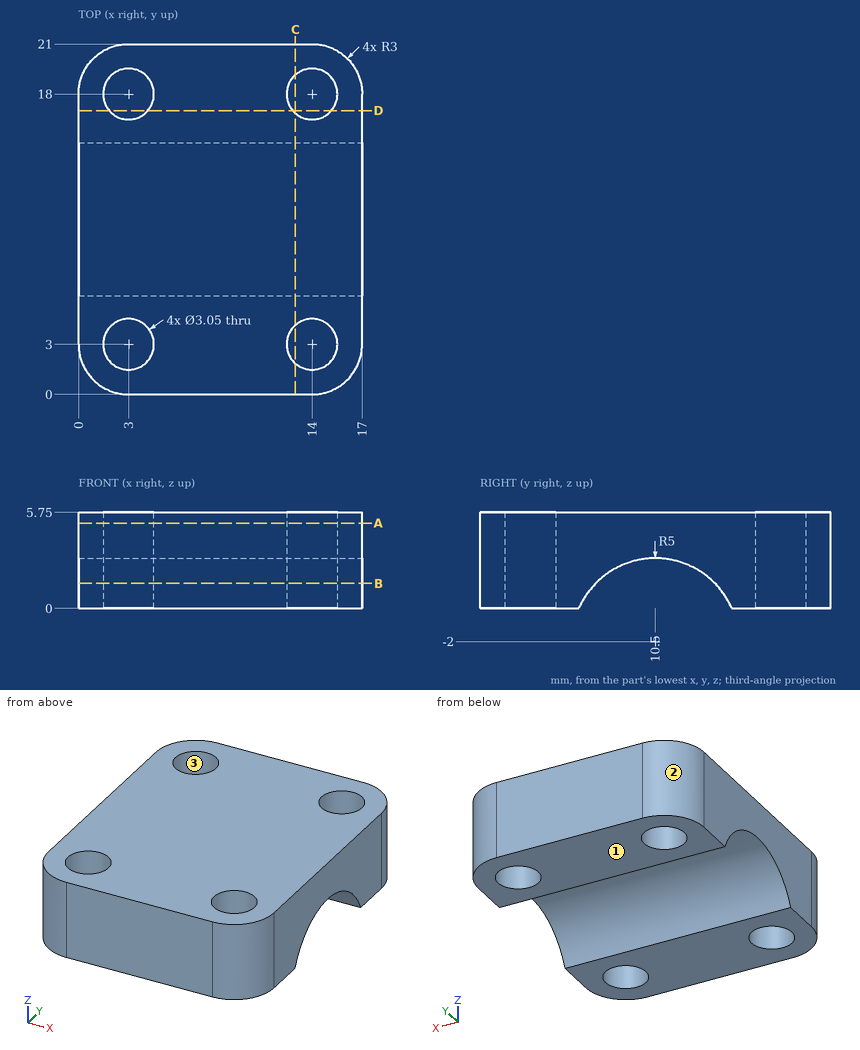
Drawing for the job (mm, zero at the part's lowest x, y, z). Give positions to 0.01 mm unless a question says otherwise; leave off trailing zeros. Write each loop counter-clockwise with the first axis right and the second up, starting at its lowest first coordinate (ties: lowest second). Pieces come first, ordered by that corner, then holes. Notation, with made-up numbers: M 77.25,70.25 L 114.25,70.25 A4 ccw 114.25,75.25 Z; hole C -14,88.5 d9. An arc over 180 degrees is marked long. Use CSV: the item, a comma, the result in double quotes.
Item 1: Slice it at A-A on z = 5.1. Write the cut outline in (x, y) (3 decimals), plus the area to 3 significant figures.
Taken from the geometry:
outline,"M 0,3 A3 ccw 3,0 L 14,0 A3 ccw 17,3 L 17,18 A3 ccw 14,21 L 3,21 A3 ccw 0,18 Z; hole C 3,3 d3.05; hole C 3,18 d3.05; hole C 14,3 d3.05; hole C 14,18 d3.05"
area,"320 mm²"
Item 2: Slice it at C-C on x = 13. Write the cut outline in (y, z), plus the area to 3 significant figures.
Taken from the geometry:
outline,"M 0,0 L 1.85,0 L 1.85,5.75 L 0,5.75 Z; M 4.15,0 L 5.92,0 A5 cw 15.08,0 L 16.85,0 L 16.85,5.75 L 4.15,5.75 Z; M 19.15,0 L 21,0 L 21,5.75 L 19.15,5.75 Z"
area,"74.5 mm²"
Item 3: Slice it at D-D on y = 17. Write the cut outline in (x, z).
Taken from the geometry:
outline,"M 0,0 L 1.85,0 L 1.85,5.75 L 0,5.75 Z; M 4.15,0 L 12.85,0 L 12.85,5.75 L 4.15,5.75 Z; M 15.15,0 L 17,0 L 17,5.75 L 15.15,5.75 Z"
Item 4: Pull direction X, two halves, no side cores. Call the marked faces 1, 2 and 3: +X half, -X half, draft (parallel to the pull), parting line (faces both ways), or undercut.
Taken from the geometry:
face 1,"draft"
face 2,"-X half"
face 3,"undercut"
Item 5: Slice it at B-B on z = 1.5. Write the cut outline in (x, y) (3 decimals).
Taken from the geometry:
outline,"M 0,3 A3 ccw 3,0 L 14,0 A3 ccw 17,3 L 17,6.929 L 0,6.929 Z; M 0,14.071 L 17,14.071 L 17,18 A3 ccw 14,21 L 3,21 A3 ccw 0,18 Z; hole C 3,3 d3.05; hole C 3,18 d3.05; hole C 14,3 d3.05; hole C 14,18 d3.05"
Item 6: Drill centre lines: probe 1 along Y at (x, z) = (14, 3.85) (3 decimals); probe 2 along Y at (x, z) = (13.75, 2); probe 3 along X at (y, z) = (18.5, 0.85). Where is each one in solid material? Low to high.
Taken from the geometry:
probe 1,"y = 0 to 1.475, 4.525 to 16.475, 19.525 to 21"
probe 2,"y = 0 to 1.5, 4.5 to 7.5, 13.5 to 16.5, 19.5 to 21"
probe 3,"x = 0.04 to 1.56, 4.44 to 12.56, 15.44 to 16.96"
Item 7: Pin check, flat tip, straight feed: P1, Ø2.5, axis at x = 3, y = 3, coming from the -Z side. Stop position of the tip, or through.
Taken from the geometry:
P1,"passes through"
